Part model, mm, in its own coordinate system. Face numbers are marked on the shaded views. Round coordinates to 2 decimals unless told otherwise and drop trailing zeros. Loops run counter-clockwise (first coordinate to the right, second up) from the corner with the lowest first, then second, coordinate; pieces in that order, holes last. Notation, with made-up numbers: (33, -20.75) -> (62, -20.75) arc R27 ccw to (62, 12.25) -> close; hole circle Ø8 at (52.25, -7). An arc over 180 degrees is marked (long way). Use a Markdown table: item, result. Add a question column.
Item 1: Two-plate mould, pull along Y, no slides. Class the marked faces 1, 2 and 3: pulls with the +Y half, pulls with the -Y half, needs draft (parallel to the pull), parting line crosses it, or undercut.
Item 2: Flat gauge pins, fed straight in: pin 1 (2.5 mm diameter, centred on x = 74.5, y = 37.5, fed in from +Z); pin 2 (12 mm diameter, centred on x = 50, z = 27.5, fed in from -Y); pin 3 (10 mm diameter, centred on x = 43, z = 44.5, fed in from -Y); pin 4 (2.5 mm diameter, centred on x = 31.75, y = 182.5, fed in from -Z). Where does each tip first touch, or does it go through?
Item 3: Cut at D-D, the plane x = 9.5. List the corners of the cut face in (y, z).
Item 4: Cut at B-B, the plane x = 74. List the corners of the cut face in (y, z).
Item 5: Cut at A-A, the plane z = 23. List the corners of the cut face in (x, y), plus the area to 3 significant figures.
Item 6: Cut at C-C, the plane x = 59. List the corners of the cut face in (y, z), plus the area to 3 significant figures.
Item 7: Probe line 1 (Y direction, x = 31.75, z = 0.25); line 2 (Z direction, x = 113, y = 32); line 3 (Y direction, x = 113, z = 36). List the from-to ranges inside material, lowest first. Write a range as [from, to].
```python
from build123d import *

# Parameters (mm, degrees)
SKETCH1_W                    = 113.5
SKETCH1_H                    = 215
BOSS_EXTRUDE1_DEPTH          = 50
CUT_EXTRUDE1_DEPTH           = 1
CUT_EXTRUDE2_DEPTH           = 1
CUT_EXTRUDE3_DEPTH           = 1
CUT_EXTRUDE4_DEPTH           = 1
CUT_EXTRUDE5_DEPTH           = 1
CUT_EXTRUDE6_DEPTH           = 1
CUT_EXTRUDE7_DEPTH           = 1
CUT_EXTRUDE8_DEPTH           = 1
CUT_EXTRUDE9_DEPTH           = 1
SKETCH11_W                   = 109.5
SKETCH11_H                   = 40
CUT_EXTRUDE10_DEPTH          = 18
CUT_EXTRUDE11_DEPTH          = 1
CUT_EXTRUDE12_DEPTH          = 1
SKETCH14_W                   = 10
SKETCH14_H                   = 18
CUT_EXTRUDE13_DEPTH          = 1
CUT_EXTRUDE14_DEPTH          = 1
F_4_0_4_DIAMETER_HOLE1_D     = 4
F_4_0_4_DIAMETER_HOLE1_DEPTH = 1
F_4_0_4_DIAMETER_HOLE2_D     = 4
F_4_0_4_DIAMETER_HOLE2_DEPTH = 1
F_4_0_4_DIAMETER_HOLE3_D     = 4
F_4_0_4_DIAMETER_HOLE3_DEPTH = 1
M48_CLEARANCE_HOLE1_D        = 56
M48_CLEARANCE_HOLE1_DEPTH    = 1
RIB1_START                   = -44
RIB1_OUTLINE_W               = 15
RIB1_OUTLINE_H               = 17
RIB1_DEPTH                   = 88


# Read off the part's stored shape, not the designer's step: Rib1
with BuildPart() as part:
    # Sketch1 → Boss-Extrude1 (new body)
    with BuildSketch(Plane.XY.offset(50)):
        with Locations((56.75, 107.5)):
            Rectangle(SKETCH1_W, SKETCH1_H)
    extrude(amount=-BOSS_EXTRUDE1_DEPTH)

    # Sketch2 → Cut-Extrude1 (cut)
    with BuildSketch(Plane.XY.offset(50)):
        with BuildLine():
            Line((18.25, 36.5), (45.25, 36.5))
            ThreePointArc((45.25, 36.5), (46.75, 38), (45.25, 39.5))
            Line((45.25, 39.5), (18.25, 39.5))
            ThreePointArc((18.25, 39.5), (16.75, 38), (18.25, 36.5))
        make_face()
    extrude(amount=-CUT_EXTRUDE1_DEPTH, mode=Mode.SUBTRACT)

    # Sketch3 → Cut-Extrude2 (cut)
    with BuildSketch(Plane.XY.offset(50)):
        with BuildLine():
            Line((18.25, 30.5), (45.25, 30.5))
            ThreePointArc((45.25, 30.5), (46.75, 32), (45.25, 33.5))
            Line((45.25, 33.5), (18.25, 33.5))
            ThreePointArc((18.25, 33.5), (16.75, 32), (18.25, 30.5))
        make_face()
    extrude(amount=-CUT_EXTRUDE2_DEPTH, mode=Mode.SUBTRACT)

    # Sketch4 → Cut-Extrude3 (cut)
    with BuildSketch(Plane.XY.offset(50)):
        with BuildLine():
            Line((18.25, 48.5), (45.25, 48.5))
            ThreePointArc((45.25, 48.5), (46.75, 50), (45.25, 51.5))
            Line((45.25, 51.5), (18.25, 51.5))
            ThreePointArc((18.25, 51.5), (16.75, 50), (18.25, 48.5))
        make_face()
    extrude(amount=-CUT_EXTRUDE3_DEPTH, mode=Mode.SUBTRACT)

    # Sketch5 → Cut-Extrude4 (cut)
    with BuildSketch(Plane.XY.offset(50)):
        with BuildLine():
            Line((18.25, 42.5), (45.25, 42.5))
            ThreePointArc((45.25, 42.5), (46.75, 44), (45.25, 45.5))
            Line((45.25, 45.5), (18.25, 45.5))
            ThreePointArc((18.25, 45.5), (16.75, 44), (18.25, 42.5))
        make_face()
    extrude(amount=-CUT_EXTRUDE4_DEPTH, mode=Mode.SUBTRACT)

    # Sketch6 → Cut-Extrude5 (cut)
    with BuildSketch(Plane.XY.offset(50)):
        with BuildLine():
            Line((68.25, 54.5), (95.25, 54.5))
            ThreePointArc((95.25, 54.5), (96.75, 56), (95.25, 57.5))
            Line((95.25, 57.5), (68.25, 57.5))
            ThreePointArc((68.25, 57.5), (66.75, 56), (68.25, 54.5))
        make_face()
    extrude(amount=-CUT_EXTRUDE5_DEPTH, mode=Mode.SUBTRACT)

    # Sketch7 → Cut-Extrude6 (cut)
    with BuildSketch(Plane.XY.offset(50)):
        with BuildLine():
            Line((18.25, 54.5), (45.25, 54.5))
            ThreePointArc((45.25, 54.5), (46.75, 56), (45.25, 57.5))
            Line((45.25, 57.5), (18.25, 57.5))
            ThreePointArc((18.25, 57.5), (16.75, 56), (18.25, 54.5))
        make_face()
    extrude(amount=-CUT_EXTRUDE6_DEPTH, mode=Mode.SUBTRACT)

    # Sketch8 → Cut-Extrude7 (cut)
    with BuildSketch(Plane.XY.offset(50)):
        with BuildLine():
            Line((68.25, 48.5), (95.25, 48.5))
            ThreePointArc((95.25, 48.5), (96.75, 50), (95.25, 51.5))
            Line((95.25, 51.5), (68.25, 51.5))
            ThreePointArc((68.25, 51.5), (66.75, 50), (68.25, 48.5))
        make_face()
    extrude(amount=-CUT_EXTRUDE7_DEPTH, mode=Mode.SUBTRACT)

    # Sketch9 → Cut-Extrude8 (cut)
    with BuildSketch(Plane.XY.offset(50)):
        with BuildLine():
            Line((68.25, 42.5), (95.25, 42.5))
            ThreePointArc((95.25, 42.5), (96.75, 44), (95.25, 45.5))
            Line((95.25, 45.5), (68.25, 45.5))
            ThreePointArc((68.25, 45.5), (66.75, 44), (68.25, 42.5))
        make_face()
    extrude(amount=-CUT_EXTRUDE8_DEPTH, mode=Mode.SUBTRACT)

    # Sketch10 → Cut-Extrude9 (cut)
    with BuildSketch(Plane.XY.offset(50)):
        with BuildLine():
            Line((68.25, 36.5), (95.25, 36.5))
            ThreePointArc((95.25, 36.5), (96.75, 38), (95.25, 39.5))
            Line((95.25, 39.5), (68.25, 39.5))
            ThreePointArc((68.25, 39.5), (66.75, 38), (68.25, 36.5))
        make_face()
    extrude(amount=-CUT_EXTRUDE9_DEPTH, mode=Mode.SUBTRACT)

    # Sketch11 → Cut-Extrude10 (cut)
    with BuildSketch(Plane.XZ):
        with Locations((56.75, 30)):
            Rectangle(SKETCH11_W, SKETCH11_H)
    extrude(amount=-CUT_EXTRUDE10_DEPTH, mode=Mode.SUBTRACT)

    # Sketch12 → Cut-Extrude11 (cut)
    with BuildSketch(Plane.XY.offset(50)):
        with BuildLine():
            Line((68.25, 30.5), (95.25, 30.5))
            ThreePointArc((95.25, 30.5), (96.75, 32), (95.25, 33.5))
            Line((95.25, 33.5), (68.25, 33.5))
            ThreePointArc((68.25, 33.5), (66.75, 32), (68.25, 30.5))
        make_face()
    extrude(amount=-CUT_EXTRUDE11_DEPTH, mode=Mode.SUBTRACT)

    # Sketch13 → Cut-Extrude12 (cut)
    with BuildSketch(Plane(origin=(113.5, 0, 0), x_dir=(0, 0, -1), z_dir=(1, 0, 0))):
        with BuildLine():
            Line((-36, 101), (-14, 101))
            ThreePointArc((-14, 101), (-12.5, 102.5), (-14, 104))
            Line((-14, 104), (-36, 104))
            ThreePointArc((-36, 104), (-37.5, 102.5), (-36, 101))
        make_face()
    extrude(amount=-CUT_EXTRUDE12_DEPTH, mode=Mode.SUBTRACT)

    # Sketch14 → Cut-Extrude13 (cut)
    with BuildSketch(Plane(origin=(113.5, 0, 0), x_dir=(0, 0, -1), z_dir=(1, 0, 0))):
        with Locations((-16, 127.5)):
            Rectangle(SKETCH14_W, SKETCH14_H)
    extrude(amount=-CUT_EXTRUDE13_DEPTH, mode=Mode.SUBTRACT)

    # Sketch15 → Cut-Extrude14 (cut)
    with BuildSketch(Plane(origin=(113.5, 0, 0), x_dir=(0, 0, -1), z_dir=(1, 0, 0))):
        with BuildLine():
            Line((-36, 94), (-14, 94))
            ThreePointArc((-14, 94), (-12.5, 95.5), (-14, 97))
            Line((-14, 97), (-36, 97))
            ThreePointArc((-36, 97), (-37.5, 95.5), (-36, 94))
        make_face()
    extrude(amount=-CUT_EXTRUDE14_DEPTH, mode=Mode.SUBTRACT)

    # Ø4.0 (4) Diameter Hole1
    with Locations(Plane(origin=(0, 0, 0), x_dir=(-1, 0, 0), z_dir=(0, 0, -1))):
        with Locations((-31.75, 182.5), (-81.75, 182.5), (-31.75, 32.5), (-81.75, 32.5)):
            Hole(F_4_0_4_DIAMETER_HOLE1_D / 2, depth=F_4_0_4_DIAMETER_HOLE1_DEPTH)

    # Ø4.0 (4) Diameter Hole2
    with Locations(Plane.ZY):
        with Locations((11.5, 32.5), (11.5, 182.5)):
            Hole(F_4_0_4_DIAMETER_HOLE2_D / 2, depth=F_4_0_4_DIAMETER_HOLE2_DEPTH)

    # Ø4.0 (4) Diameter Hole3
    with Locations(Plane(origin=(113.5, 0, 0), x_dir=(0, 0, -1), z_dir=(1, 0, 0))):
        with Locations((-36.5, 32.5), (-11.5, 32.5), (-36.5, 182.5), (-11.5, 182.5)):
            Hole(F_4_0_4_DIAMETER_HOLE3_D / 2, depth=F_4_0_4_DIAMETER_HOLE3_DEPTH)

    # M48 Clearance Hole1
    with Locations(Plane.XY.offset(50)):
        with Locations((35, 167)):
            Hole(M48_CLEARANCE_HOLE1_D / 2, depth=M48_CLEARANCE_HOLE1_DEPTH)

    # Rib1 outline → Rib1 (add)
    with BuildSketch(Plane(origin=(62.5, 0, 0), x_dir=(0, 0, -1), z_dir=(1, 0, 0)).offset(RIB1_START)):
        with Locations((-17.5, 9.5)):
            Rectangle(RIB1_OUTLINE_W, RIB1_OUTLINE_H)
    extrude(amount=RIB1_DEPTH)


solid = part.part
```
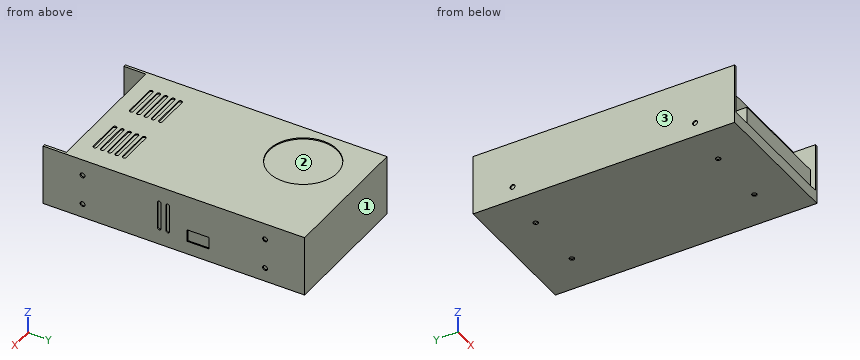
A:
| question | item | result |
|---|---|---|
| 1 | face 1 | pulls with the +Y half |
| 1 | face 2 | undercut |
| 1 | face 3 | needs draft |
| 2 | pin 1 | stops at z = 50 |
| 2 | pin 2 | stops at y = 1 |
| 2 | pin 3 | stops at y = 18 |
| 2 | pin 4 | stops at z = 1 |
| 3 | outline | (0, 0) -> (215, 0) -> (215, 50) -> (178.57, 50) -> (178.57, 49) -> (155.43, 49) -> (155.43, 50) -> (18, 50) -> (18, 10) -> (0, 10) -> close |
| 4 | outline | (0, 0) -> (215, 0) -> (215, 50) -> (57.5, 50) -> (57.5, 49) -> (54.5, 49) -> (54.5, 50) -> (51.5, 50) -> (51.5, 49) -> (48.5, 49) -> (48.5, 50) -> (45.5, 50) -> (45.5, 49) -> (42.5, 49) -> (42.5, 50) -> (39.5, 50) -> (39.5, 49) -> (36.5, 49) -> (36.5, 50) -> (33.5, 50) -> (33.5, 49) -> (30.5, 49) -> (30.5, 50) -> (18, 50) -> (18, 25) -> (1, 25) -> (1, 10) -> (0, 10) -> close |
| 5 | outline | (0, 0) -> (2, 0) -> (2, 18) -> (18.5, 18) -> (18.5, 1) -> (106.5, 1) -> (106.5, 18) -> (111.5, 18) -> (111.5, 0) -> (113.5, 0) -> (113.5, 94) -> (112.5, 94) -> (112.5, 97) -> (113.5, 97) -> (113.5, 101) -> (112.5, 101) -> (112.5, 104) -> (113.5, 104) -> (113.5, 215) -> (0, 215) -> close |
| 5 | area | 23,900 mm^2 |
| 6 | outline | (0, 0) -> (215, 0) -> (215, 50) -> (181.42, 50) -> (181.42, 49) -> (152.58, 49) -> (152.58, 50) -> (18, 50) -> (18, 25) -> (1, 25) -> (1, 10) -> (0, 10) -> close |
| 6 | area | 10,300 mm^2 |
| 7 | line 1 | y = [0, 30.5], [34.5, 180.5], [184.5, 215] |
| 7 | line 2 | z = [0, 9.56], [13.44, 34.56], [38.44, 50] |
| 7 | line 3 | y = [0, 30.56], [34.44, 94], [97, 101], [104, 180.56], [184.44, 215] |
